from build123d import *

# Parameters (mm, degrees)
F0_W        = 41.8725572526
F0_H        = 24.7696824372
F1_DEPTH    = 63.5
F3_D        = 11.43
F4_C1_SIZE2 = 5.08
F4_C1_SIZE  = 2.54
F4_C2_SIZE2 = 2.54
F4_C2_SIZE  = 5.08
F4_C3_SIZE2 = 5.08
F4_C3_SIZE  = 2.54
F4_C4_SIZE2 = 2.54
F4_C4_SIZE  = 5.08
F5_R        = 5.08
F6_T1_DEPTH = 42.5496824372
F6_T3_DEPTH = 79.1980633142
F7_T1_DEPTH = 42.5496824372
F7_T3_DEPTH = 79.1980633142


# Not quite as in the source:
# - a fillet or chamfer that OpenCascade refuses, or shapes differently, is made with other operations: its cross-section is extruded or revolved along the edge and cut away or added


with BuildPart() as f1:
    # F0 (on Top) → F1 (new body)
    with BuildSketch(Plane.XY):
        with Locations((20.9362786263, 12.3848412186)):
            Rectangle(F0_W, F0_H)
    extrude(amount=F1_DEPTH)

    # F3 (through all)
    with Locations(Plane.XY.offset(63.5)):
        with Locations((20.6414014101, 12.7780102193)):
            Hole(F3_D / 2)

    # F4: chamfer of 2.54 x 5.08 on 4 edges, made by hand

    # F4_c1
    f4_c1_edges = [f1.edges().sort_by_distance(p)[0] for p in [
        (0, 24.7696824372, 31.75),
    ]]
    f4_c1_side = f1.faces().sort_by_distance((0, 24.7188824372, 31.75))[0]
    chamfer(f4_c1_edges, length=F4_C1_SIZE, length2=F4_C1_SIZE2, reference=f4_c1_side)

    # F4_c2
    f4_c2_edges = [f1.edges().sort_by_distance(p)[0] for p in [
        (41.8725572526, 24.7696824372, 31.75),
    ]]
    f4_c2_side = f1.faces().sort_by_distance((41.8217572526, 24.7696824372, 31.75))[0]
    chamfer(f4_c2_edges, length=F4_C2_SIZE, length2=F4_C2_SIZE2, reference=f4_c2_side)

    # F4_c3
    f4_c3_edges = [f1.edges().sort_by_distance(p)[0] for p in [
        (20.9362786263, 24.7696824372, 0),
    ]]
    f4_c3_side = f1.faces().sort_by_distance((20.9362786263, 24.7188824372, 0))[0]
    chamfer(f4_c3_edges, length=F4_C3_SIZE, length2=F4_C3_SIZE2, reference=f4_c3_side)

    # F4_c4
    f4_c4_edges = [f1.edges().sort_by_distance(p)[0] for p in [
        (20.9362786263, 24.7696824372, 63.5),
    ]]
    f4_c4_side = f1.faces().sort_by_distance((20.9362786263, 24.7696824372, 63.4492))[0]
    chamfer(f4_c4_edges, length=F4_C4_SIZE, length2=F4_C4_SIZE2, reference=f4_c4_side)

    # F5
    f5_edges = [f1.edges().sort_by_distance(p)[0] for p in [
        (0, 0, 31.75),
        (41.872557, 0, 31.75),
        (20.936279, 0, 0),
        (20.936279, 0, 63.5),
    ]]
    fillet(f5_edges, radius=F5_R)

    # F6: fillet of radius 5.08 on 4 edges, made by hand

    # F6_s2 → F6_t1 (cut)
    with BuildSketch(Plane.XZ.offset(-34.9296824372)):
        with BuildLine():
            ThreePointArc((5.08, 0), (1.4878975516, 1.4878975516), (0, 5.08))
            Line((0, 5.08), (0, 0))
            Line((0, 0), (5.08, 0))
        make_face()
        with BuildLine():
            ThreePointArc((5.08, 63.5), (1.4878975516, 62.0121024484), (0, 58.42))
            Line((0, 58.42), (0, 63.5))
            Line((0, 63.5), (5.08, 63.5))
        make_face()
    extrude(amount=F6_T1_DEPTH, mode=Mode.SUBTRACT)

    # F6_s4 → F6_t3 (cut)
    with BuildSketch(Plane.XY.offset(-7.8490316571)):
        with BuildLine():
            ThreePointArc((0, 19.0900697743), (0.7586938936, 21.7607838239), (2.8081549349, 23.6337599046))
            Line((2.8081549349, 23.6337599046), (0, 22.2296824372))
            Line((0, 22.2296824372), (0, 19.0900697743))
        make_face()
    extrude(amount=F6_T3_DEPTH, mode=Mode.SUBTRACT)

    # F7: fillet of radius 5.08 on 4 edges, made by hand

    # F7_s2 → F7_t1 (cut)
    with BuildSketch(Plane.XZ.offset(-34.9296824372)):
        with BuildLine():
            ThreePointArc((41.8725572526, 5.08), (40.3846597011, 1.4878975516), (36.7925572526, 0))
            Line((36.7925572526, 0), (41.8725572526, 0))
            Line((41.8725572526, 0), (41.8725572526, 5.08))
        make_face()
        with BuildLine():
            ThreePointArc((41.8725572526, 58.42), (40.3846597011, 62.0121024484), (36.7925572526, 63.5))
            Line((36.7925572526, 63.5), (41.8725572526, 63.5))
            Line((41.8725572526, 63.5), (41.8725572526, 58.42))
        make_face()
    extrude(amount=F7_T1_DEPTH, mode=Mode.SUBTRACT)

    # F7_s4 → F7_t3 (cut)
    with BuildSketch(Plane.XY.offset(-7.8490316571)):
        with BuildLine():
            ThreePointArc((41.8725572526, 19.0900697743), (41.1138633591, 21.7607838239), (39.0644023178, 23.6337599046))
            Line((39.0644023178, 23.6337599046), (41.8725572526, 22.2296824372))
            Line((41.8725572526, 22.2296824372), (41.8725572526, 19.0900697743))
        make_face()
    extrude(amount=F7_T3_DEPTH, mode=Mode.SUBTRACT)


solid = f1.part
For this review, take the finished solid that the model builds, in its own axes (mm). Round coordinates to 2 decimals unless told otherwise and drop trailing zeros. Write each loop counter-clockwise with the first axis right and the second up, starting at its lowest first coordinate (ties: lowest second). Pieces come first, ordered by that corner, then holes. Notation, with made-up numbers: M 57.25,5.5 L 84.25,5.5 A22 cw 84.25,26.5 Z; hole C -25,-40 d9. An arc over 180 degrees is marked long. Write item = value, one per line. Start each with the question number.
(1) We need section B-B (y = 9.75). Give the boundary of the cut face in (x, z).
(2) The part is to be moulded in two halves that separate along X. For faces 1 (the face through (21.385, 18.444, 31.305)), 2 (the face through (41.873, 12, 31)), 3 (the face through (20.67, 23.52, 2.58)), say which applies: +X half, -X half, draft (parallel to the pull), parting line (faces both ways), or undercut.
(3) For line 1 along X through (y, z) = (13, 57.5); line 2 along Y through (x, z) = (20.5, 50); line 3 along X through (y, z) = (7.75, 25), list the stretches that pass through material, from the lowest coordinate up.
(4) We need section C-C (z = 18). Give the boundary of the cut face in (x, y) (3 decimals), then the cut area to 3 significant figures.
(5) We need section D-D (x = 29). Give the boundary of the cut face in (y, z), then the cut area to 3 significant figures.
(6) We need section A-A (x = 17). Give the boundary of the cut face in (y, z).
Results found:
q1.outline = M 0,5.08 A5.08 ccw 5.08,0 L 15.79,0 L 15.79,63.5 L 5.08,63.5 A5.08 ccw 0,58.42 Z; M 25.49,0 L 36.79,0 A5.08 ccw 41.87,5.08 L 41.87,58.42 A5.08 ccw 36.79,63.5 L 25.49,63.5 Z
q2.face_1 = undercut
q2.face_2 = +X half
q2.face_3 = draft
q3.line_1 = 0 to 14.93, 26.35 to 41.87
q3.line_2 = 0 to 7.06, 18.49 to 24.77
q3.line_3 = 0 to 17.92, 23.36 to 41.87
q4.outline = M 0,5.08 A5.08 ccw 5.08,0 L 36.793,0 A5.08 ccw 41.873,5.08 L 41.873,19.09 A5.08 ccw 39.064,23.634 L 36.793,24.77 L 5.08,24.77 L 2.808,23.634 A5.08 ccw 0,19.09 Z; hole C 20.641,12.778 d11.43
q4.area = 907 mm²
q5.outline = M 0,5.08 A5.08 ccw 5.08,0 L 22.23,0 L 24.77,5.08 L 24.77,58.42 L 22.23,63.5 L 5.08,63.5 A5.08 ccw 0,58.42 Z
q5.area = 1,550 mm²
q6.outline = M 0,5.08 A5.08 ccw 5.08,0 L 8.37,0 L 8.37,63.5 L 5.08,63.5 A5.08 ccw 0,58.42 Z; M 17.18,0 L 22.23,0 L 24.77,5.08 L 24.77,58.42 L 22.23,63.5 L 17.18,63.5 Z
